Work out the finished part from the listing and answer in its coordinate system (mm). A direction names the side the tool comes from. Coordinates: 2 decimals unless noted, no trailing zeros. Write each loop counter-clockwise with the first axis right and the second up, starting at its lowest first coordinate (ties: lowest second). Pieces come first, ordered by that corner, then holes. Notation, with made-up numbers: (5.25, 83) - (39.25, 83) arc R16 cw to (39.25, 89) - close; hole circle Ø8 at (-7.75, 8). An arc over 180 degrees is marked (long way). Answer as a JSON object with one key per item and string values. Group by question number.
from build123d import *

# Parameters (mm, degrees)
SKETCH_1_W      = 40
SKETCH_1_H      = 20
EXTRUDE_1_DEPTH = 36
SKETCH_2_W      = 1.671860453
SKETCH_2_H      = 20
EXTRUDE_2_DEPTH = 10
SKETCH_5_W      = 1.442469022
SKETCH_5_H      = 19.996010925
EXTRUDE_5_DEPTH = 10
SKETCH_7_R      = 6.5
EXTRUDE_6_DEPTH = 2


with BuildPart() as part:
    # 草图1 → 凸台-拉伸1 (new body)
    with BuildSketch(Plane.XY):
        with Locations((-345.403508772, -241.771929825)):
            Rectangle(SKETCH_1_W, SKETCH_1_H)
    extrude(amount=-EXTRUDE_1_DEPTH)

    # 草图2 → 凸台-拉伸2 (add)
    with BuildSketch(Plane(origin=(-365.403508772, 0, -0.001996536), x_dir=(0, 0, 1), z_dir=(-1, 0, 0))):
        with Locations((-25.87591575, -241.714058127)):
            Rectangle(SKETCH_2_W, SKETCH_2_H)
    extrude(amount=EXTRUDE_2_DEPTH)

    # 草图5 → 凸台-拉伸5 (add)
    with BuildSketch(Plane(origin=(-325.403508772, 0, -0.752936531), x_dir=(0, 0, -1), z_dir=(1, 0, 0))):
        with Locations((24.676802168, -241.807464448)):
            Rectangle(SKETCH_5_W, SKETCH_5_H)
    extrude(amount=EXTRUDE_5_DEPTH)

    # 草图7 → 凸台-拉伸6 (add)
    with BuildSketch(Plane(origin=(-2.226236695, -0.840173037, -36), x_dir=(-1, 0, 0), z_dir=(0, 0, -1))):
        with Locations(Location((333.308396358, -240.749438329, 0), (0, 0, 180))):
            Circle(SKETCH_7_R)
    extrude(amount=EXTRUDE_6_DEPTH)


solid = part.part
Q1. Section D-D on y = -246 is taken. Determine the outline of the cut face in (x, z).
Q2. A tool of negligible diameter and unlimited length cuts with its end or side. For faces 1 (the face through (-329.53, -239.1, -36.99)), 2 (the face through (-320, -242, -26.151)), 3 (the face through (-320, -231.809, -25)), from which of +Z, -Z, +X, -X, +Y, -Y can it reach the whole face along a straight path? Write none if from no direction.
Q3. Section A-A on y = -234.25 is taken. Determine the outline of the cut face in (x, z).
Q4. Section C-C on z = -30.5 is taken. Determine the outline of the cut face in (x, y), plus the area to 3 significant figures.
Q5. Consider L1, parallel to Y at x = -353, z = -31; L2, parallel to Z at x = -344, y = -238.5; L3, parallel to X at y = -232.5, z = -3.5. Determine where each line is inside the solid, lowest interval first. Write a range as from..to.
Q6. Section B-B on x = -338.5 is taken. Determine the outline of the cut face in (y, z).
Q7. Flat-ended cylindrical pins translate along their axes: pin 1 Ø5 at (x, y) = (-371.5, -239) entering from +Z; pin 2 Ø1.5 at (x, z) = (-338, -19.5) entering from -Y; pin 3 Ø2 at (x, y) = (-326, -246) entering from -Z. Find the tip coordinate at first contact, or state that the pin passes through.
Numbers:
{
 "1": {"outline": "(-375.4, -26.71) - (-365.4, -26.71) - (-365.4, -36) - (-340.31, -36) - (-340.31, -38) - (-330.76, -38) - (-330.76, -36) - (-325.4, -36) - (-325.4, -26.15) - (-315.4, -26.15) - (-315.4, -24.71) - (-325.4, -24.71) - (-325.4, 0) - (-365.4, 0) - (-365.4, -25.04) - (-375.4, -25.04) - close"},
 "2": {"face 1": "-Z", "face 2": "-Z, +X, +Y, -Y", "face 3": "+Z, -Z, +X, +Y"},
 "3": {"outline": "(-375.4, -26.71) - (-365.4, -26.71) - (-365.4, -36) - (-325.4, -36) - (-325.4, -26.15) - (-315.4, -26.15) - (-315.4, -24.71) - (-325.4, -24.71) - (-325.4, 0) - (-365.4, 0) - (-365.4, -25.04) - (-375.4, -25.04) - close"},
 "4": {"outline": "(-365.4, -251.77) - (-325.4, -251.77) - (-325.4, -231.77) - (-365.4, -231.77) - close", "area": "800 mm²"},
 "5": {"L1": "y = -251.77..-231.77", "L2": "z = -36..0", "L3": "x = -365.4..-325.4"},
 "6": {"outline": "(-251.77, -36) - (-247.37, -36) - (-247.37, -38) - (-235.81, -38) - (-235.81, -36) - (-231.77, -36) - (-231.77, 0) - (-251.77, 0) - close"},
 "7": {"pin 1": "stops at z = -25.04", "pin 2": "stops at y = -251.77", "pin 3": "stops at z = -36"}
}
